Source: CAD feature listing. Evaluate the final solid. Frame: model axes, mm. Face numbers are marked on the shaded views. A direction names the side the tool comes from. Round coordinates to 2 decimals unless told otherwise and drop trailing zeros. Loops run counter-clockwise (first coordinate to the right, second up) from the corner with the lowest first, then second, coordinate; pieces in that order, holes last. Notation, with made-up numbers: M 35.5,30.5 L 49.5,30.5 A15 cw 49.5,46.5 Z; hole C -38.5,33.5 d7. An arc over 180 degrees is marked long. Answer as a JSON object with one key per item and string values.
from build123d import *

# Parameters (mm, degrees)
BOSS_EXTRUDE1_DEPTH = 76.2
SKETCH3_R           = 6.35
CUT_EXTRUDE1_DEPTH  = 76.2
SKETCH4_R           = 6.35
CUT_EXTRUDE2_DEPTH  = 76.2
SKETCH5_R           = 22.225
SKETCH5_R_2         = 4.7625
CUT_EXTRUDE3_DEPTH  = 76.2


with BuildPart() as part:
    # Sketch2 → Boss-Extrude1 (new body)
    with BuildSketch(Plane(origin=(0, 0, 0), x_dir=(0, 0, -1), z_dir=(1, 0, 0))):
        Polygon((-78.818556701, -25.334536082), (86.281443299, -25.334536082), (86.281443299, -50.734536082), (98.981443299, -50.734536082), (98.981443299, -25.334536082), (98.981443299, -12.634536082), (-66.118556701, -12.634536082), (-66.118556701, 12.765463918), (-78.818556701, 12.765463918), (-78.818556701, -6.875900942), align=None)
    extrude(amount=BOSS_EXTRUDE1_DEPTH)

    # Sketch3 → Cut-Extrude1 (cut)
    with BuildSketch(Plane(origin=(0, 0, -98.981443299), x_dir=(-1, 0, 0), z_dir=(0, 0, -1))):
        with Locations((-57.15, -38.034536082)):
            Circle(SKETCH3_R)
        with Locations((-19.05, -38.034536082)):
            Circle(SKETCH3_R)
    extrude(amount=-CUT_EXTRUDE1_DEPTH, mode=Mode.SUBTRACT)

    # Sketch4 → Cut-Extrude2 (cut)
    with BuildSketch(Plane(origin=(0, 0, 66.118556701), x_dir=(-1, 0, 0), z_dir=(0, 0, -1))):
        with Locations((-57.15, 0.065463918)):
            Circle(SKETCH4_R)
        with Locations((-19.05, 0.065463918)):
            Circle(SKETCH4_R)
    extrude(amount=-CUT_EXTRUDE2_DEPTH, mode=Mode.SUBTRACT)

    # Sketch5 → Cut-Extrude3 (cut)
    with BuildSketch(Plane(origin=(0, -12.634536082, 0), x_dir=(1, 0, 0), z_dir=(0, 1, 0))):
        with Locations((38.1, 10.081443299)):
            Circle(SKETCH5_R)
        with Locations((38.1, 54.531443299)):
            Circle(SKETCH5_R_2)
        with Locations((38.1, -34.368556701)):
            Circle(SKETCH5_R_2)
    extrude(amount=-CUT_EXTRUDE3_DEPTH, mode=Mode.SUBTRACT)


solid = part.part
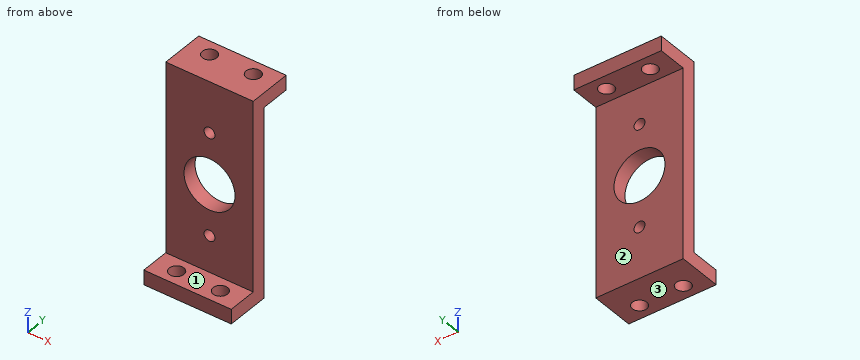
Item 1: Section C-C on x = 49. Return the cut outline in (y, z), then the cut area to 3 significant figures.
Answer sheet:
{"outline": "M -50.73,-98.98 L -12.63,-98.98 L -12.63,-29.45 L -25.33,-29.45 L -25.33,-86.28 L -50.73,-86.28 Z; M -25.33,9.29 L -12.63,9.29 L -12.63,66.12 L 12.77,66.12 L 12.77,78.82 L -25.33,78.82 Z", "area": "2,410 mm²"}
Item 2: Section D-D on z = -72. Return the cut outline in (x, y).
Answer sheet:
{"outline": "M 0,-25.33 L 76.2,-25.33 L 76.2,-12.63 L 0,-12.63 Z"}
Item 3: Contact query for flat-ended pins moving along their axis: pin 1 Ø10 at (x, y) = (25.5, -37.5) entering from +Z; pin 2 Ø6 at (x, y) = (67.5, -10) entering from -Z; pin 3 Ø4 at (x, z) = (21.5, -63.5) entering from -Y; pin 4 Ø5 at (x, z) = (18, -71) entering from +Y. Output: stop coordinate, or through.
Answer sheet:
{"pin 1": "stops at z = -86.28", "pin 2": "stops at z = -98.98", "pin 3": "stops at y = -25.33", "pin 4": "stops at y = -12.63"}
Item 4: Access query for the marked faces 1, 2 and 3. Directions: +Z, -Z, +X, -X, +Y, -Y. A direction counts if a zero-diameter tool reaches every point of the face in a straight line with its end or side. Return the directions, or none.
Answer sheet:
{"face 1": "+Z, +X, -X, -Y", "face 2": "-Z, +X, -X, +Y", "face 3": "-Z, +X, -X, +Y, -Y"}
Item 5: Section B-B on y = -3. Return the cut outline in (x, z).
Answer sheet:
{"outline": "M 0,66.12 L 13.49,66.12 L 13.49,78.82 L 0,78.82 Z; M 24.61,66.12 L 51.59,66.12 L 51.59,78.82 L 24.61,78.82 Z; M 62.71,66.12 L 76.2,66.12 L 76.2,78.82 L 62.71,78.82 Z"}
Item 6: Line query: probe 1 along Z at (x, y) = (38.1, -17.5); probe 2 along X at (y, z) = (2, 71); probe 3 along Y at (x, z) = (24.5, -85). Output: solid intervals per line, ascending. Write a range as from..to.
Answer sheet:
{"probe 1": "z = -98.98..-59.29, -49.77..-32.31, 12.14..29.61, 39.13..78.82", "probe 2": "x = 0..13, 25.1..51.1, 63.2..76.2", "probe 3": "y = -25.33..-12.63"}
Item 7: Section A-A on x = 38.1. Return the cut outline in (y, z), then the cut area to 3 significant figures.
Answer sheet:
{"outline": "M -50.73,-98.98 L -12.63,-98.98 L -12.63,-59.29 L -25.33,-59.29 L -25.33,-86.28 L -50.73,-86.28 Z; M -25.33,-49.77 L -12.63,-49.77 L -12.63,-32.31 L -25.33,-32.31 Z; M -25.33,12.14 L -12.63,12.14 L -12.63,29.61 L -25.33,29.61 Z; M -25.33,39.13 L -12.63,39.13 L -12.63,66.12 L 12.77,66.12 L 12.77,78.82 L -25.33,78.82 Z", "area": "2,100 mm²"}
